Source: CAD feature listing. Evaluate the final solid. Frame: model axes, mm. A direction names the side the tool comes from. Give positions to 0.01 mm unless a question says otherwise; leave off trailing zeros. Order: outer loops, then holes, each group sorted by start corner. A loop starts at its lowest first (then second) coordinate and runs counter-clockwise, first axis right, second up.
1) Section A-A, the plane x = 0. Return loops of the section in (y, z).
2) Material intervals for line 1 (Z direction, x = 0, y = 1.55); line 2 (X direction, y = 1.25, z = -12); line 3 (Z direction, x = 0.5, y = 3), sorted ascending.
3) Access query for faces 1 (the face through (-4, 2, 0)), 2 (the face through (2.86, 11.89, 0.9)). Directions: +Z, -Z, +X, -X, +Y, -Y. A direction counts if a zero-diameter tool reaches every point of the face in a straight line with its end or side. Return the directions, or none.
4) Section B-B, the plane z = 0. Return loops of the section in (x, y).
5) First-contact query: P1, Ø4, axis at x = -2.5, y = 17.5, coming from the -Z side; P2, Ø1.5, axis at x = 2.5, y = 5.5, coming from the -Z side; P3, Ø1, axis at y = 12.5, z = -1.5, coming from the -X side. Flat tips, straight axial feed; report the tip coordinate or a pass-through.
6) Section C-C, the plane y = 2. Return loops of the section in (x, z), plus the area to 3 significant figures.
7) Section D-D, the plane x = 2.5. Return loops of the section in (y, z).
8) Draft query along X for faces 3 (the face through (0, 0, 0)), 4 (the face through (0, 2, -16)), 5 (the face through (1.2, 2, 10.4)). Return one class per face: released by +X, released by -X, zero draft, split by the parting line, or undercut.
Autodesk Inventor part; units mm, degrees
ref_plane "YZ Plane" through (0, 0, 0) normal (1, 0, 0) x (0, 1, 0)
ref_plane "XZ Plane" through (0, 0, 0) normal (0, 1, 0) x (-1, 0, 0)
ref_plane "XY Plane" through (0, 0, 0) normal (0, 0, 1) x (1, 0, 0)
sketch "Sketch1" plane through (0, 0, 0) normal (0, 1, 0) x (-1, 0, 0)
  line L0 (0, 12) -> (0, -12) construction
  line L1 (-4, 12) -> (-4, -12)
  line L2 (4, -12) -> (4, 12)
  arc A0 (4, 12) -> (-4, 12) centre (0, 12) ccw
  arc A1 (-4, -12) -> (4, -12) centre (0, -12) ccw
  point P0 (0, 0)
  point P1 (0, 0)
  dimension "d0" = 24
  dimension "d1" = 8
extrude "Extrusion1" add sketch "Sketch1" along normal blind 4
sketch "Sketch2" plane through (0, 4, 0) normal (0, 1, 0) x (1, 0, 0)
  circle A0 centre (0, 0) radius 3
  dimension "d4" = 6
extrude "Extrusion2" add sketch "Sketch2" along normal blind 16
sketch "Sketch3" plane through (0, 0, 0) normal (1, 0, 0) x (0, 1, 0)
  circle A0 centre (15, 0) radius 1
  line L0 (20, -3) -> (20, 3)
  point P0 (0, 0)
  dimension "d7" = 2
  dimension "d8" = 5
extrude "Extrusion3" cut sketch "Sketch3" along normal mid plane 16
sketch "Sketch4" plane through (0, 4, 0) normal (0, 1, 0) x (1, 0, 0)
  arc A0 (4, 12) -> (-4, 12) centre (0, 12) ccw
  arc A1 (-4, -12) -> (4, -12) centre (0, -12) ccw
hole "Hole1" at (0, 4, 12) at (0, 4, -12) direction (0, -1, 0) diameter 4 end through all
properties part number "Crank"
From the geometry:
1. outline: (0, -16) - (4, -16) - (4, -14) - (0, -14) - close; (0, -10) - (4, -10) - (4, -3) - (20, -3) - (20, 3) - (4, 3) - (4, 10) - (0, 10) - close; (0, 14) - (4, 14) - (4, 16) - (0, 16) - close; hole circle Ø2 at (15, 0)
2. line 1: z = -16 to -14, -10 to 10, 14 to 16
2. line 2: x = -4 to -2, 2 to 4
2. line 3: z = -15.97 to -13.94, -10.06 to 10.06, 13.94 to 15.97
3. face 1: +Z, -Z, -X, +Y, -Y
3. face 2: +Y
4. outline: (-4, 0) - (4, 0) - (4, 4) - (3, 4) - (3, 14) - (-3, 14) - (-3, 4) - (-4, 4) - close; (-3, 16) - (3, 16) - (3, 20) - (-3, 20) - close
5. P1: stops at z = -2.96
5. P2: stops at z = -2.44
5. P3: stops at x = -2.83
6. outline: (-4, -12) arc R4 ccw to (4, -12) - (4, 12) arc R4 ccw to (-4, 12) - close; hole circle Ø4 at (0, -12); hole circle Ø4 at (0, 12)
6. area: 217 mm2
7. outline: (0, -15.12) - (4, -15.12) - (4, -1.66) - (20, -1.66) - (20, 1.66) - (4, 1.66) - (4, 15.12) - (0, 15.12) - close; hole circle Ø2 at (15, 0)
8. face 3: zero draft
8. face 4: split by the parting line
8. face 5: undercut
